Input: dimensioned drawing with shaded views. Units: mm. Origin: part minimum x, y, z. Coordinates: 2 decimals unless noted, no trailing zeros. Loops run counter-clockwise (first coordinate to the right, second up) from the corner with the lowest first, then second, coordinate; pieces in that order, holes last.
Item 1: Pin query (flat end, axial travel): pin 1 Ø5 at (x, y) = (6.5, 29.5) entering from +Z; pin 2 Ø5 at (x, z) = (40, 19.51) entering from -Y; pin 3 Ø4 at (x, y) = (26, 15) entering from -Z; pin 4 Ø4 at (y, z) = (57, 26) entering from +X. Return the tip coordinate at first contact, or that it passes through.
Item 2: Pull-direction query (X, two-part tool) for the marked faces 1, 2 and 3; classes: +X half, -X half, draft (parallel to the pull), parting line (faces both ways), or undercut.
Item 3: Section query A-A, the plane x = 32.5. Return the cut outline in (y, z).
Item 4: Section query D-D, the plane x = 58. Return the cut outline in (y, z).
Item 5: Section query B-B, the plane y = 9.5. Return the cut outline in (x, z), then the cut area to 3 significant figures.
Item 6: Section query C-C, the plane z = 58. Return the cut outline in (x, y).
Item 7: Line query: probe 1 along X at (y, z) = (68.7, 32.5); probe 2 along Z at (x, y) = (25, 66); probe 3 along Y at (x, z) = (39, 11.5). Output: solid intervals per line, ascending.
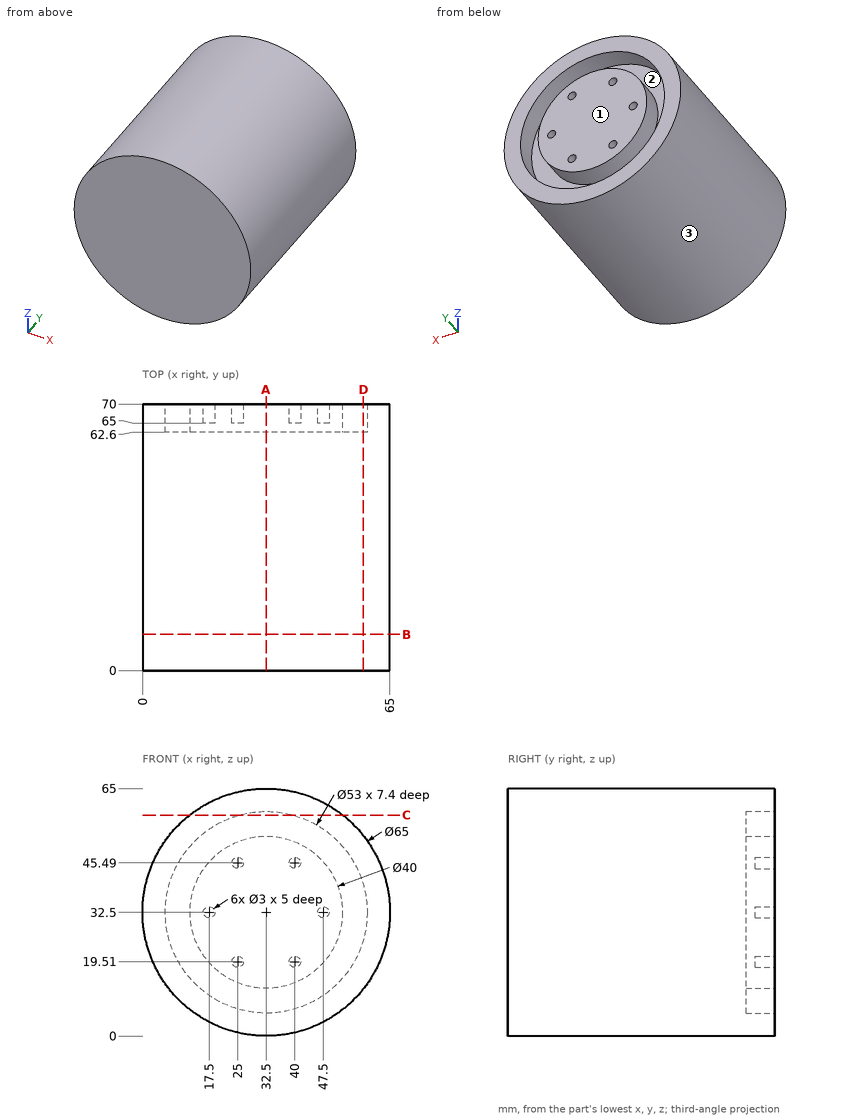
Verdict:
1. pin 1: stops at z = 54.95
1. pin 2: stops at y = 0
1. pin 3: stops at z = 0.31
1. pin 4: stops at x = 64.69
2. face 1: draft
2. face 2: undercut
2. face 3: parting line
3. outline: (0, 0) - (70, 0) - (70, 6) - (62.6, 6) - (62.6, 12.5) - (70, 12.5) - (70, 52.5) - (62.6, 52.5) - (62.6, 59) - (70, 59) - (70, 65) - (0, 65) - close
4. outline: (0, 12.35) - (70, 12.35) - (70, 25.29) - (62.6, 25.29) - (62.6, 39.71) - (70, 39.71) - (70, 52.65) - (0, 52.65) - close
5. outline: circle Ø65 at (32.5, 32.5)
5. area: 3,320 mm2
6. outline: (12.35, 0) - (52.65, 0) - (52.65, 70) - (39.71, 70) - (39.71, 62.6) - (25.29, 62.6) - (25.29, 70) - (12.35, 70) - close
7. probe 1: x = 0 to 6, 12.5 to 16, 19 to 46, 49 to 52.5, 59 to 65
7. probe 2: z = 0.88 to 7.08, 13.96 to 18.01, 21.01 to 43.99, 46.99 to 51.04, 57.92 to 64.12
7. probe 3: y = 0 to 62.6
